Build history of the part. All positions in model axes, mm. Face numbers are marked on the shaded views. A direction names the side the tool comes from. Coordinates: 2 decimals unless noted, no trailing zeros. Loops run counter-clockwise (first coordinate to the right, second up) from the corner with the lowest first, then second, coordinate; pieces in that order, holes last.
(1) Wall check: L1, parallel to Y at x = -2.75, z = 2; L2, parallel to X at y = 0.5, z = 0; L3, parallel to Z at x = -1.75, y = 2. Give the ranges that are in metal, low to high.
(2) Slice it at A-A (x = 0). Give the cut face in (y, z).
(3) Slice it at C-C (y = 5.5). Give the cut face in (x, z).
(4) Flat gauge pins, fed straight in: P1, Ø4, axis at y = 1, z = -4, coming from the +X side; P2, Ø1.5, axis at x = -2.5, y = 1, coming from the -Z side. Where does each tip first touch, or does it go through?
(5) Slice it at D-D (z = 3). Give the cut face in (x, y), and give its area (3 significant figures).
(6) Slice it at B-B (z = 0). Give the cut face in (x, y), and give its area (3 significant figures).
(7) Tool access for the marked faces 1 and 2: list every direction of +Z, -Z, +X, -X, +Y, -Y with a clear straight run to the whole face (end or side of a thin tool).
from build123d import *

# Parameters (mm, degrees)
SKETCH1_R           = 2.55
BOSS_EXTRUDE1_DEPTH = 7
SKETCH1_3_R         = 5.5
SKETCH1_3_R_2       = 2.55
BOSS_EXTRUDE2_DEPTH = 1
FILLET1_R           = 1


with BuildPart() as part:
    # Sketch1 → Boss-Extrude1 (new body)
    with BuildSketch(Plane(origin=(0, 0, 0), x_dir=(1, 0, 0), z_dir=(0, 1, 0))):
        Circle(SKETCH1_R)
    extrude(amount=BOSS_EXTRUDE1_DEPTH)

    # Sketch1_3 → Boss-Extrude2 (add)
    with BuildSketch(Plane(origin=(0, 0, 0), x_dir=(1, 0, 0), z_dir=(0, 1, 0))):
        Circle(SKETCH1_3_R)
        Circle(SKETCH1_3_R_2, mode=Mode.SUBTRACT)
        Circle(SKETCH1_3_R_2)
    extrude(amount=-BOSS_EXTRUDE2_DEPTH)

    # Fillet1
    fillet1_edges = [part.edges().sort_by_distance(p)[0] for p in [
        (-2.55, 7, 0),
    ]]
    fillet(fillet1_edges, radius=FILLET1_R)


solid = part.part
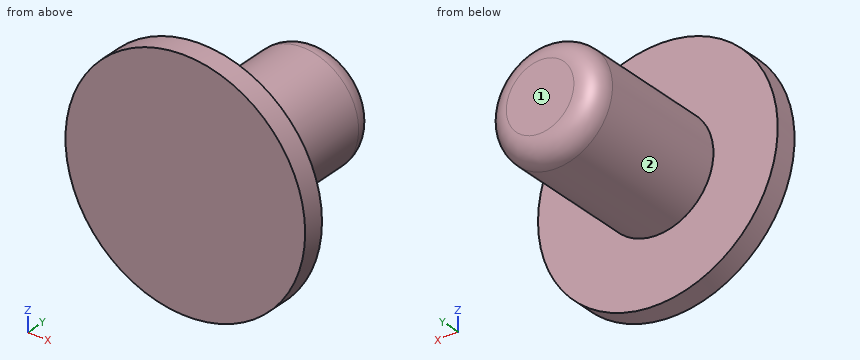
Response values:
1. L1: y = -1 to 0
1. L2: x = -2.55 to 2.55
1. L3: z = -1.85 to 1.85
2. outline: (-1, -5.5) - (0, -5.5) - (0, -2.55) - (6, -2.55) arc R1 ccw to (7, -1.55) - (7, 1.55) arc R1 ccw to (6, 2.55) - (0, 2.55) - (0, 5.5) - (-1, 5.5) - close
3. outline: circle Ø5.1 at (0, 0)
4. P1: stops at x = 5.01
4. P2: stops at z = -1.85
5. outline: (-4.61, -1) - (4.61, -1) - (4.61, 0) - (-4.61, 0) - close
5. area: 9.22 mm2
6. outline: (-5.5, -1) - (5.5, -1) - (5.5, 0) - (2.55, 0) - (2.55, 6) arc R1 ccw to (1.55, 7) - (-1.55, 7) arc R1 ccw to (-2.55, 6) - (-2.55, 0) - (-5.5, 0) - close
6. area: 46.3 mm2
7. face 1: +Z, -Z, +X, -X, +Y
7. face 2: +Y
